Can you work these out from the model? Positions are in its coordinate system, mm. Give positions to 0.01 mm unless a question says otherwise; leave off trailing zeros. Loops run counter-clockwise (first coordinate to the right, second up) from the corner with the lowest first, then second, coordinate; pieces in that order, holes last. Notation, with made-up numbers: (58, -23) -> (87, -23) arc R19 cw to (87, -6) -> close; hole circle Ø7 at (9.5, 6.5). An arc over 180 degrees is marked (long way). Return JSON: item names as keys, results as strings. Group by question number.
Q1. Suppose I cut it at B-B, the plane y = -6. Please give me the cut outline in (x, z).
Q2. Will these pins go through, and if not, where does the flat tip stop? pin 1 (6 mm diameter, centred on x = -8, y = -11, fed in from -Z); pin 2 (0.8 mm diameter, centred on y = -3, z = 1, fed in from -X).
Q3. Suppose I cut it at C-C, the plane y = 13. Please give me the cut outline in (x, z), and give its area (3 significant figures).
Q4. Suppose I cut it at A-A, the plane z = 1.2. Please give me the cut outline in (x, y), and give its area (3 significant figures).
Q5. Suppose I cut it at D-D, the plane x = -5. Please give me the cut outline in (y, z).
Q6. I need wall thicknesses on line 1 along Y through (x, z) = (-10, 1.05); line 2 along X through (y, z) = (0, 0.75); line 3 along Y through (x, z) = (5, 1.35). Which ranges of each line are inside material? Lowest first, please. Write a range as [from, to].
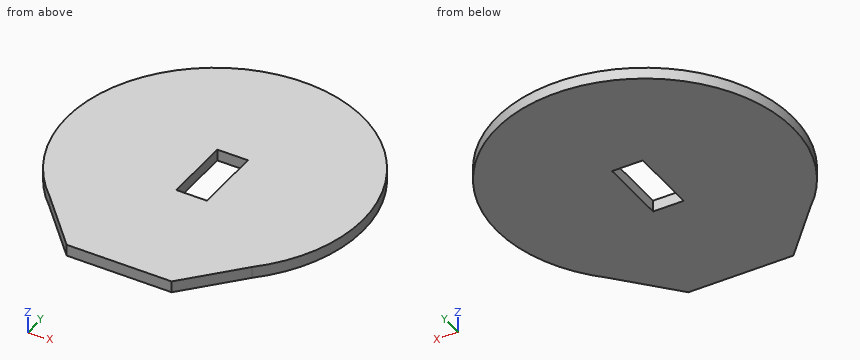
```python
from build123d import *

# Parameters (mm, degrees)
BOSS_EXTRUDE1_DEPTH = 1.5
CUT_EXTRUDE1_REACH  = 38.943
SKETCH2_W           = 4
SKETCH2_H           = 9


with BuildPart() as part:
    # Sketch1 → Boss-Extrude1 (new body)
    with BuildSketch(Plane.XY):
        with BuildLine():
            Line((-17.310520711, -21.823889376), (-3.597740248, -21.843555797))
            Line((-3.597740248, -21.843555797), (2.757908107, -14.842465178))
            ThreePointArc((2.757908107, -14.842465178), (-10.455115829, 18.525441507), (-23.668139764, -14.842465178))
            Line((-23.668139764, -14.842465178), (-17.310520711, -21.823889376))
        make_face()
    extrude(amount=BOSS_EXTRUDE1_DEPTH)

    # Sketch2 → Cut-Extrude1 (cut, up to next)
    with BuildSketch(Plane.XY.offset(1.5), mode=Mode.PRIVATE) as cut_extrude1_sk1:
        with Locations((-10.090473375, -2.029514736)):
            Rectangle(SKETCH2_W, SKETCH2_H)
    cut_extrude1_tool1 = extrude(cut_extrude1_sk1.sketch, amount=-CUT_EXTRUDE1_REACH, mode=Mode.PRIVATE) & part.part
    add(cut_extrude1_tool1.solids().sort_by_distance((-10.090473, -2.029515, 1.5))[0], mode=Mode.SUBTRACT)


solid = part.part
```
Ans:
{
 "1": {"outline": "(-29.03, 0) -> (-12.09, 0) -> (-12.09, 1.5) -> (-29.03, 1.5) -> close; (-8.09, 0) -> (8.12, 0) -> (8.12, 1.5) -> (-8.09, 1.5) -> close"},
 "2": {"pin 1": "stops at z = 0", "pin 2": "stops at x = -29.67"},
 "3": {"outline": "(-23.97, 0) -> (3.06, 0) -> (3.06, 1.5) -> (-23.97, 1.5) -> close", "area": "40.6 mm^2"},
 "4": {"outline": "(-23.67, -14.84) -> (-17.31, -21.82) -> (-3.6, -21.84) -> (2.76, -14.84) arc R19.3 ccw (long way) to start; hole (-12.09, -6.53) -> (-8.09, -6.53) -> (-8.09, 2.47) -> (-12.09, 2.47) -> close", "area": "1,180 mm^2"},
 "5": {"outline": "(-21.84, 0) -> (17.74, 0) -> (17.74, 1.5) -> (-21.84, 1.5) -> close"},
 "6": {"line 1": "y = [-21.83, -6.53], [2.47, 18.52]", "line 2": "x = [-29.74, -12.09], [-8.09, 8.83]", "line 3": "y = [-12.33, 10.79]"}
}
